from build123d import *

# Parameters (mm, degrees)
BOSS_EXTRUDE1_DEPTH = 5
BOSS_EXTRUDE2_DEPTH = 18


with BuildPart() as part:
    # Sketch1 → Boss-Extrude1 (new body)
    with BuildSketch(Plane.XY):
        with BuildLine():
            Line((40, 0), (4.437851134, 0))
            ThreePointArc((4.437851134, 0), (4.745844393, -0.956791275), (4.85, -1.956521739))
            ThreePointArc((4.85, -1.956521739), (4.745844393, -2.956252203), (4.437851134, -3.913043478))
            Line((4.437851134, -3.913043478), (40, -3.913043478))
            Line((40, -3.913043478), (40, -3.806521739))
            ThreePointArc((40, -3.806521739), (38.15, -1.956521739), (40, -0.106521739))
            Line((40, -0.106521739), (40, 0))
        make_face()
    extrude(amount=BOSS_EXTRUDE1_DEPTH)

    # Sketch1_3 → Boss-Extrude2 (add)
    with BuildSketch(Plane.XY):
        with BuildLine():
            Line((0, -3.913043478), (0, 0))
            Line((0, 0), (4.437851134, 0))
            ThreePointArc((4.437851134, 0), (-4.85, -1.956521739), (4.437851134, -3.913043478))
            Line((4.437851134, -3.913043478), (0, -3.913043478))
        make_face()
        with BuildLine():
            Line((4.437851134, 0), (0, 0))
            Line((0, 0), (0, -3.913043478))
            Line((0, -3.913043478), (4.437851134, -3.913043478))
            ThreePointArc((4.437851134, -3.913043478), (4.745844393, -2.956252203), (4.85, -1.956521739))
            ThreePointArc((4.85, -1.956521739), (4.745844393, -0.956791275), (4.437851134, 0))
        make_face()
        with BuildLine():
            ThreePointArc((41.85, -1.956521739), (41.308147545, -0.648374194), (40, -0.106521739))
            Line((40, -0.106521739), (40, -3.806521739))
            ThreePointArc((40, -3.806521739), (41.308147545, -3.264669284), (41.85, -1.956521739))
        make_face()
        with BuildLine():
            Line((40, -3.806521739), (40, -0.106521739))
            ThreePointArc((40, -0.106521739), (38.15, -1.956521739), (40, -3.806521739))
        make_face()
    extrude(amount=BOSS_EXTRUDE2_DEPTH)


solid = part.part
CAD build for the part. Positions are in the model's coordinates, mm. A direction names the side the tool comes from. Coordinates: 2 decimals unless noted, no trailing zeros. Loops run counter-clockwise (first coordinate to the right, second up) from the corner with the lowest first, then second, coordinate; pieces in that order, holes last. Notation, with made-up numbers: (83.5, -34) - (125.5, -34) arc R34 cw to (125.5, -1) - close; hole circle Ø10 at (83.25, 26.5). An arc over 180 degrees is marked (long way). Use one line per item in the form item = value. Start each with the question number.
1) Band-saw the part on D-D (y = 0.5). Give the cut face in (x, z).
2) Two-plate mould, pull along X, no slides. Class faces 1 (the face through (22, -2, 5)), 2 (the face through (40, -2, 18)): +X half, -X half, draft (parallel to the pull), parting line (faces both ways), or undercut.
3) Band-saw the part on C-C (x = 22). Give the cut face in (y, z), and give its area (3 significant figures).
4) Tool access for faces 3 (the face through (22, 0, 2)), 4 (the face through (22, -3.913, 2)), 5 (the face through (13, -2, 0)): list every direction of +Z, -Z, +X, -X, +Y, -Y with a clear straight run to the whole face (end or side of a thin tool).
5) Band-saw the part on A-A (z = 16.25). Give the cut face in (x, y).
6) Drill centre lines: L1, parallel to Z at x = 30.5, y = -3.25; L2, parallel to Y at x = 31.5, z = 4; L3, parallel to X at y = -3.5, z = 16. Where is each one in solid material? Low to high. Write a range as from..to.
7) Flat gauge pins, fed straight in: pin 1 (5.5 mm diameter, centred on x = 22.5, z = 3, fed in from -Y); pin 2 (4 mm diameter, centred on x = 8, y = -1, fed in from +Z); pin 3 (3 mm diameter, centred on y = -4.5, z = 13, fed in from -X). Where does each tip first touch, or does it go through?
8) Band-saw the part on B-B (z = 2.25). Give the cut face in (x, y).
Check values:
q1.outline = (-4.18, 0) - (4.18, 0) - (4.18, 18) - (-4.18, 18) - close
q2.face_1 = undercut
q2.face_2 = draft
q3.outline = (-3.91, 0) - (0, 0) - (0, 5) - (-3.91, 5) - close
q3.area = 19.6 mm2
q4.face_3 = +Z, -Z, +X, +Y
q4.face_4 = +Z, -Z, +X, -Y
q4.face_5 = -Z, +X, -X, +Y, -Y
q5.outline = circle Ø9.7 at (0, -1.96); circle Ø3.7 at (40, -1.96)
q6.L1 = 0..5
q6.L2 = -3.91..0
q6.L3 = -4.6..4.6, 38.98..41.02
q7.pin_1 = -3.91
q7.pin_2 = 5
q7.pin_3 = -4.74
q8.outline = (4.44, -3.91) - (40, -3.91) - (40, -3.81) arc R1.85 ccw to (40, -0.11) - (40, 0) - (4.44, 0) arc R4.85 ccw (long way) to start
